```python
from build123d import *

# Parameters (mm, degrees)
F0_R     = 10.5
F1_DEPTH = 3.5
F2_R     = 5
F3_DEPTH = 1
F4_R     = 4.1
F5_DEPTH = 3
F6_SIZE2 = 2
F6_SIZE  = 3


with BuildPart() as f1:
    # F0 (on Top) → F1 (new body)
    with BuildSketch(Plane.XY):
        Circle(F0_R)
    extrude(amount=F1_DEPTH)

    # F2 (on face) → F3 (join)
    with BuildSketch(Plane.XY.offset(3.5)):
        Circle(F2_R)
    extrude(amount=F3_DEPTH)

    # F4 (on face) → F5 (join)
    with BuildSketch(Plane.XY.offset(4.5)):
        Circle(F4_R)
    extrude(amount=F5_DEPTH)

    # F6
    f6_edges = [f1.edges().sort_by_distance(p)[0] for p in [
        (-10.5, 0, 3.5),
    ]]
    f6_side = f1.faces().sort_by_distance((-10.203015, 0, 3.5))[0]
    chamfer(f6_edges, length=F6_SIZE, length2=F6_SIZE2, reference=f6_side)


solid = f1.part
```
The listing builds one solid part. Answer for the finished solid, in the listing's coordinates (mm). A direction names the side the tool comes from. Coordinates: 2 decimals unless noted, no trailing zeros. Loops run counter-clockwise (first coordinate to the right, second up) from the corner with the lowest first, then second, coordinate; pieces in that order, holes last. Notation, with made-up numbers: M 86.25,26.5 L 114.25,26.5 A23 cw 114.25,39.5 Z; hole C -13,-16 d4. An arc over 180 degrees is marked long. Answer as a JSON object with one key per item and string values. Group by question number.
Item 1: Each of these flat-tipped pins is pushed along its axis until it touches: P1, Ø3, axis at x = -8, y = 7, coming from the +Z side; P2, Ø4, axis at x = 3, z = 4, coming from the -Y side. Where does it stop, or does it pass through?
Item 2: Section C-C (z = 1) is taken. Write down the section's boundary in (x, y).
Item 3: Consider L1, parallel to Z at x = 1.75, y = 5; L2, parallel to X at y = -2.5, z = 2.5; L3, parallel to Z at x = -9.25, y = 1.5. Determine where each line is inside the solid, lowest interval first.
Item 4: Which of the six approach directions +Z, -Z, +X, -X, +Y, -Y give full straight-line access (tool end or side, diameter ignored) to faces 1 (the face through (0, 0, 0)), 2 (the face through (5, -2, 3.5))?
Item 5: Section D-D (z = 6.5) is taken. Write down the section's boundary in (x, y).
Item 6: Section A-A (x = 0) is taken. Write down the section's boundary in (y, z).
Solved:
{
 "1": {"P1": "stops at z = 2.41", "P2": "stops at y = -9.33"},
 "2": {"outline": "C 0,0 d21"},
 "3": {"L1": "z = 0 to 3.5", "L2": "x = -8.65 to 8.65", "L3": "z = 0 to 2.25"},
 "4": {"face 1": "-Z, +X, -X, +Y, -Y", "face 2": "+Z"},
 "5": {"outline": "C 0,0 d8.2"},
 "6": {"outline": "M -10.5,0 L 10.5,0 L 10.5,1.5 L 7.5,3.5 L 5,3.5 L 5,4.5 L 4.1,4.5 L 4.1,7.5 L -4.1,7.5 L -4.1,4.5 L -5,4.5 L -5,3.5 L -7.5,3.5 L -10.5,1.5 Z"}
}
